```python
from build123d import *

# Parameters (mm, degrees)
SKETCH1_W            = 50.2
SKETCH1_H            = 5
BOSS_EXTRUDE1_DEPTH  = 26.2
SKETCH2_W            = 45.2
SKETCH2_H            = 23.699783527
CUT_EXTRUDE1_DEPTH   = 26.2
SKETCH4_W            = 1.5
SKETCH4_H            = 24.2
CUT_EXTRUDE2_DEPTH   = 26.2
SKETCH5_W            = 2
SKETCH5_H            = 5
BOSS_EXTRUDE2_DEPTH  = 3
SKETCH7_W            = 1.5
SKETCH7_H            = 24.2
CUT_EXTRUDE3_DEPTH   = 23
SKETCH8_W            = 45.2
SKETCH8_H            = 1.5
CUT_EXTRUDE4_DEPTH   = 23
SKETCH9_W            = 2
SKETCH9_H            = 5
BOSS_EXTRUDE3_DEPTH  = 3
SKETCH11_W           = 2
SKETCH11_H           = 5
BOSS_EXTRUDE4_DEPTH  = 2
SKETCH12_W           = 2
SKETCH12_H           = 4.997290344
BOSS_EXTRUDE5_DEPTH  = 2
SKETCH15_W           = 1
SKETCH15_H           = 5
BOSS_EXTRUDE6_DEPTH  = 4.65
SKETCH16_W           = 1
SKETCH16_H           = 5
BOSS_EXTRUDE7_DEPTH  = 4.65
SKETCH17_W           = 1
SKETCH17_H           = 5
BOSS_EXTRUDE8_DEPTH  = 9
SKETCH18_W           = 1
SKETCH18_H           = 5
BOSS_EXTRUDE9_DEPTH  = 9
SKETCH20_W           = 10
SKETCH20_H           = 5
BOSS_EXTRUDE10_DEPTH = 2
SKETCH21_W           = 10
SKETCH21_H           = 5
BOSS_EXTRUDE11_DEPTH = 2
SKETCH22_W           = 23.2
SKETCH22_H           = 5
BOSS_EXTRUDE12_DEPTH = 3
SKETCH23_W           = 23.2
SKETCH23_H           = 5
BOSS_EXTRUDE13_DEPTH = 3
SKETCH24_W           = 54.5
SKETCH24_H           = 5
BOSS_EXTRUDE14_DEPTH = 3
SKETCH25_W           = 3
SKETCH25_H           = 5
BOSS_EXTRUDE15_DEPTH = 3
SKETCH26_W           = 3
SKETCH26_H           = 5
BOSS_EXTRUDE16_DEPTH = 3
SKETCH27_W           = 13
SKETCH27_H           = 5
BOSS_EXTRUDE17_DEPTH = 3
SKETCH28_W           = 13
SKETCH28_H           = 5
BOSS_EXTRUDE18_DEPTH = 3
SKETCH29_W           = 2
SKETCH29_H           = 5
BOSS_EXTRUDE21_DEPTH = 10
SKETCH30_W           = 2
SKETCH30_H           = 4.997290344
BOSS_EXTRUDE22_DEPTH = 10
SKETCH31_W           = 13.5
SKETCH31_H           = 5
BOSS_EXTRUDE23_DEPTH = 2
SKETCH32_W           = 13.5
SKETCH32_H           = 5
BOSS_EXTRUDE24_DEPTH = 2
SKETCH33_R           = 1.6
CUT_EXTRUDE5_DEPTH   = 12
SKETCH34_R           = 1.6
CUT_EXTRUDE6_DEPTH   = 12


with BuildPart() as part:
    # Sketch1 → Boss-Extrude1 (new body)
    with BuildSketch(Plane.XY):
        with Locations((-66.582634731, 11.968862275)):
            Rectangle(SKETCH1_W, SKETCH1_H)
    extrude(amount=BOSS_EXTRUDE1_DEPTH)

    # Sketch2 → Cut-Extrude1 (cut)
    with BuildSketch(Plane.XZ.offset(-9.468862275)):
        with Locations((-66.582634731, 11.849891764)):
            Rectangle(SKETCH2_W, SKETCH2_H)
    extrude(amount=-CUT_EXTRUDE1_DEPTH, mode=Mode.SUBTRACT)

    # Sketch4 → Cut-Extrude2 (cut)
    with BuildSketch(Plane.XZ.offset(-9.468862275)):
        with Locations((-90.932634731, 14.1)):
            Rectangle(SKETCH4_W, SKETCH4_H)
    extrude(amount=-CUT_EXTRUDE2_DEPTH, mode=Mode.SUBTRACT)

    # Sketch5 → Boss-Extrude2 (add)
    with BuildSketch(Plane.ZY.offset(91.682634731)):
        with Locations((1, 11.968862275)):
            Rectangle(SKETCH5_W, SKETCH5_H)
    extrude(amount=BOSS_EXTRUDE2_DEPTH)

    # Sketch7 → Cut-Extrude3 (cut)
    with BuildSketch(Plane.XZ.offset(-9.468862275)):
        with Locations((-42.232634731, 14.1)):
            Rectangle(SKETCH7_W, SKETCH7_H)
    extrude(amount=-CUT_EXTRUDE3_DEPTH, mode=Mode.SUBTRACT)

    # Sketch8 → Cut-Extrude4 (cut)
    with BuildSketch(Plane.XZ.offset(-9.468862275)):
        with Locations((-66.582634731, 24.449783527)):
            Rectangle(SKETCH8_W, SKETCH8_H)
    extrude(amount=-CUT_EXTRUDE4_DEPTH, mode=Mode.SUBTRACT)

    # Sketch9 → Boss-Extrude3 (add)
    with BuildSketch(Plane(origin=(-41.482634731, 0, 0), x_dir=(0, 0, -1), z_dir=(1, 0, 0))):
        with Locations((-1, 11.968862275)):
            Rectangle(SKETCH9_W, SKETCH9_H)
    extrude(amount=BOSS_EXTRUDE3_DEPTH)

    # Sketch11 → Boss-Extrude4 (add)
    with BuildSketch(Plane(origin=(-38.482634731, 0, 0), x_dir=(0, 0, -1), z_dir=(1, 0, 0))):
        with Locations((-1, 11.968862275)):
            Rectangle(SKETCH11_W, SKETCH11_H)
    extrude(amount=BOSS_EXTRUDE4_DEPTH)

    # Sketch15 → Boss-Extrude6 (add)
    with BuildSketch(Plane.ZY.offset(90.182634731)):
        with Locations((25.7, 11.968862275)):
            Rectangle(SKETCH15_W, SKETCH15_H)
    extrude(amount=BOSS_EXTRUDE6_DEPTH)

    # Sketch16 → Boss-Extrude7 (add)
    with BuildSketch(Plane(origin=(-42.982634731, 0, 0), x_dir=(0, 0, -1), z_dir=(1, 0, 0))):
        with Locations((-25.7, 11.968862275)):
            Rectangle(SKETCH16_W, SKETCH16_H)
    extrude(amount=BOSS_EXTRUDE7_DEPTH)

    # Sketch17 → Boss-Extrude8 (add)
    with BuildSketch(Plane.XY.offset(26.2)):
        with Locations((-38.832634731, 11.968862275)):
            Rectangle(SKETCH17_W, SKETCH17_H)
    extrude(amount=BOSS_EXTRUDE8_DEPTH)

    # Sketch18 → Boss-Extrude9 (add)
    with BuildSketch(Plane.XY.offset(26.2)):
        with Locations((-94.332634731, 11.968862275)):
            Rectangle(SKETCH18_W, SKETCH18_H)
    extrude(amount=BOSS_EXTRUDE9_DEPTH)

    # Sketch20 → Boss-Extrude10 (add)
    with BuildSketch(Plane.ZY.offset(94.832634731)):
        with Locations((30.2, 11.968862275)):
            Rectangle(SKETCH20_W, SKETCH20_H)
    extrude(amount=BOSS_EXTRUDE10_DEPTH)

    # Sketch21 → Boss-Extrude11 (add)
    with BuildSketch(Plane(origin=(-38.332634731, 0, 0), x_dir=(0, 0, -1), z_dir=(1, 0, 0))):
        with Locations((-30.2, 11.968862275)):
            Rectangle(SKETCH21_W, SKETCH21_H)
    extrude(amount=BOSS_EXTRUDE11_DEPTH)

    # Sketch22 → Boss-Extrude12 (add)
    with BuildSketch(Plane.ZY.offset(90.182634731)):
        with Locations((13.6, 11.968862275)):
            Rectangle(SKETCH22_W, SKETCH22_H)
    extrude(amount=BOSS_EXTRUDE12_DEPTH)

    # Sketch23 → Boss-Extrude13 (add)
    with BuildSketch(Plane(origin=(-42.982634731, 0, 0), x_dir=(0, 0, -1), z_dir=(1, 0, 0))):
        with Locations((-13.6, 11.968862275)):
            Rectangle(SKETCH23_W, SKETCH23_H)
    extrude(amount=BOSS_EXTRUDE13_DEPTH)

    # Sketch24 → Boss-Extrude14 (add)
    with BuildSketch(Plane.XY.offset(26.2)):
        with Locations((-66.582634731, 11.968862275)):
            Rectangle(SKETCH24_W, SKETCH24_H)
    extrude(amount=BOSS_EXTRUDE14_DEPTH)

    # Sketch25 → Boss-Extrude15 (add)
    with BuildSketch(Plane.XY.offset(35.2)):
        with Locations((-37.832634731, 11.968862275)):
            Rectangle(SKETCH25_W, SKETCH25_H)
    extrude(amount=BOSS_EXTRUDE15_DEPTH)

    # Sketch26 → Boss-Extrude16 (add)
    with BuildSketch(Plane.XY.offset(35.2)):
        with Locations((-95.332634731, 11.968862275)):
            Rectangle(SKETCH26_W, SKETCH26_H)
    extrude(amount=BOSS_EXTRUDE16_DEPTH)

    # Sketch27 → Boss-Extrude17 (add)
    with BuildSketch(Plane.ZY.offset(96.832634731)):
        with Locations((31.7, 11.968862275)):
            Rectangle(SKETCH27_W, SKETCH27_H)
    extrude(amount=BOSS_EXTRUDE17_DEPTH)

    # Sketch28 → Boss-Extrude18 (add)
    with BuildSketch(Plane(origin=(-36.332634731, 0, 0), x_dir=(0, 0, -1), z_dir=(1, 0, 0))):
        with Locations((-31.7, 11.968862275)):
            Rectangle(SKETCH28_W, SKETCH28_H)
    extrude(amount=BOSS_EXTRUDE18_DEPTH)

    # Sketch29 → Boss-Extrude21 (add)
    with BuildSketch(Plane(origin=(-36.482634731, 0, 0), x_dir=(0, 0, -1), z_dir=(1, 0, 0))):
        with Locations((-1, 11.968862275)):
            Rectangle(SKETCH29_W, SKETCH29_H)
    extrude(amount=BOSS_EXTRUDE21_DEPTH)


with BuildPart() as body_2:
    # Sketch12 → Boss-Extrude5 (new body)
    with BuildSketch(Plane.ZY.offset(94.682634731)):
        with Locations((1, 11.970217103)):
            Rectangle(SKETCH12_W, SKETCH12_H)
    extrude(amount=BOSS_EXTRUDE5_DEPTH)


    add(part.part)  # Boss-Extrude22 merges part
    # Sketch30 → Boss-Extrude22 (add)
    with BuildSketch(Plane.ZY.offset(96.682634731)):
        with Locations((1, 11.970217103)):
            Rectangle(SKETCH30_W, SKETCH30_H)
    extrude(amount=BOSS_EXTRUDE22_DEPTH)

    # Sketch31 → Boss-Extrude23 (add)
    with BuildSketch(Plane.XY.offset(2)):
        with Locations((-99.932634731, 11.968862275)):
            Rectangle(SKETCH31_W, SKETCH31_H)
    extrude(amount=BOSS_EXTRUDE23_DEPTH)

    # Sketch32 → Boss-Extrude24 (add)
    with BuildSketch(Plane.XY.offset(2)):
        with Locations((-33.232634731, 11.968862275)):
            Rectangle(SKETCH32_W, SKETCH32_H)
    extrude(amount=BOSS_EXTRUDE24_DEPTH)

    # Sketch33 → Cut-Extrude5 (cut)
    with BuildSketch(Plane.XY.offset(4)):
        with Locations((-104.419830922, 11.968862275)):
            Circle(SKETCH33_R)
    extrude(amount=-CUT_EXTRUDE5_DEPTH, mode=Mode.SUBTRACT)

    # Sketch34 → Cut-Extrude6 (cut)
    with BuildSketch(Plane.XY.offset(4)):
        with Locations((-29.31902414, 11.968862275)):
            Circle(SKETCH34_R)
    extrude(amount=-CUT_EXTRUDE6_DEPTH, mode=Mode.SUBTRACT)


solid = body_2.part
```
The model under review builds one solid part; all positions refer to its coordinate system, in mm. A direction names the side the tool comes from. Give positions to 0.01 mm unless a question says otherwise; leave off trailing zeros. Loops run counter-clockwise (first coordinate to the right, second up) from the corner with the lowest first, then second, coordinate; pieces in that order, holes last. Notation, with made-up numbers: (63.25, -26.5) - (86.25, -26.5) arc R19 cw to (86.25, -7.5) - close; hole circle Ø3 at (83.5, -18.75). An arc over 180 degrees is marked (long way). Answer as a JSON object with one key per item and string values.
Q1. Add section B-B on y = 11.2. State the section outline as (x, z) points, plus the area to 3 significant figures.
Worked out:
{"outline": "(-106.68, 0) - (-105.82, 0) - (-105.82, 4) - (-106.68, 4) - close; (-103.02, 0) - (-89.18, 0) - (-89.18, 25.2) - (-43.98, 25.2) - (-43.98, 0) - (-30.72, 0) - (-30.72, 4) - (-39.98, 4) - (-39.98, 25.2) - (-33.33, 25.2) - (-33.33, 38.2) - (-39.33, 38.2) - (-39.33, 29.2) - (-93.83, 29.2) - (-93.83, 38.2) - (-99.83, 38.2) - (-99.83, 25.2) - (-93.18, 25.2) - (-93.18, 4) - (-103.02, 4) - close; (-27.92, 0) - (-26.48, 0) - (-26.48, 4) - (-27.92, 4) - close", "area": "661 mm^2"}
Q2. Add section C-C on z = 36. State the section outline as (x, y) points, plus the area to 3 significant figures.
Worked out:
{"outline": "(-99.83, 9.47) - (-93.83, 9.47) - (-93.83, 14.47) - (-99.83, 14.47) - close; (-39.33, 9.47) - (-33.33, 9.47) - (-33.33, 14.47) - (-39.33, 14.47) - close", "area": "60.0 mm^2"}
Q3. Insertion check: pin 1 (1.9 mm diameter, centred on x = -104.42, y = 11.97, fed in from +Z); pin 2 (1.5 mm diameter, centred on y = 11.5, z = 34.5, fed in from -X); pin 3 (1.5 mm diameter, centred on x = -65, y = 11.5, fed in from -Z); pin 4 (2.5 mm diameter, centred on y = 10.5, z = 14, fed in from -X). Each pin has a flat end and moves straight along its axis. Give the tip position at first contact, or say it passes through.
Worked out:
{"pin 1": "passes through", "pin 2": "stops at x = -99.83", "pin 3": "stops at z = 25.2", "pin 4": "stops at x = -93.18"}
Q4. To check wall thickness, follow line 1 along X through (y, z) = (11.95, 3.5); line 2 along X through (y, z) = (10.9, 32); line 3 along X through (y, z) = (11, 2). State the ranges of each line that lie inside material, in increasing order.
Worked out:
{"line 1": "x = -106.68 to -106.02, -102.82 to -89.18, -43.98 to -30.92, -27.72 to -26.48", "line 2": "x = -99.83 to -93.83, -39.33 to -33.33", "line 3": "x = -106.68 to -105.69, -103.15 to -89.18, -43.98 to -30.59, -28.05 to -26.48"}
Q5. For faces 1 (the flat face through (-100, 12, 4)), 2 (the flat face through (-43.983, 12, 12)), 3 (the flat face through (-37, 12, 25.2)), 4 (the flat face through (-67, 12, 29.2)), list the 3-axis set-ups (+Z, -Z, +X, -X, +Y, -Y) from which the entire face can be reached by the end or side of a thin tool; tool diameter is ignored.
Worked out:
{"face 1": "-X, +Y, -Y", "face 2": "-Z, +Y, -Y", "face 3": "+X, +Y, -Y", "face 4": "+Z, +Y, -Y"}
Q6. Add section A-A on z = 19. State the section outline as (x, y) points, plus the area to 3 significant figures.
Worked out:
{"outline": "(-93.18, 9.47) - (-89.18, 9.47) - (-89.18, 14.47) - (-93.18, 14.47) - close; (-43.98, 9.47) - (-39.98, 9.47) - (-39.98, 14.47) - (-43.98, 14.47) - close", "area": "40.0 mm^2"}
Q7. Mouldability with a two-part tool opening along Z and no side actions: class faces 5 (the flat face through (-33, 12, 4)), 6 (the flat face through (-67, 12, 25.2)), 7 (the flat face through (-106.683, 12, 2)) as +Z half, -Z half, draft (parallel to the pull), parting line (faces both ways), or undercut.
Worked out:
{"face 5": "undercut", "face 6": "-Z half", "face 7": "draft"}
Q8. Add section D-D on x = -80. State the section outline as (y, z) points, plus the area to 3 significant figures.
Worked out:
{"outline": "(9.47, 25.2) - (14.47, 25.2) - (14.47, 29.2) - (9.47, 29.2) - close", "area": "20.0 mm^2"}
